Geometry: final body of the model. Coordinates: model frame, mm. Face numbers are marked on the shaded views. A direction names the side the tool comes from. Coordinates: 2 decimals unless noted, no trailing zeros. Loops run counter-clockwise (first coordinate to the right, second up) from the corner with the lowest first, then second, coordinate; pieces in that order, holes last. Notation, with made-up numbers: (-16.5, 26.25) - (3.5, 26.25) arc R22 cw to (3.5, 62.25) - close; hole circle Ø8 at (15, 46). An arc over 180 degrees is marked (long way). Put each result on its own line as item: value. Start each with the question number.
1) Section D-D on x = 33. Output: boundary loops of the cut face in (y, z).
2) Material intervals for line 1 along X through (y, z) = (-3, 0); line 2 along Y through (x, z) = (0, 420); line 3 along Z through (x, y) = (0, -7), sorted ascending. Write a range as from..to.
3) Section A-A on x = 0. Output: boundary loops of the cut face in (y, z).
4) Reachability of the marked faces 1, 2 and 3 from +Z, -Z, +X, -X, +Y, -Y: full face, straight path, thin tool, end or side. Return the list, or none.
5) Section C-C on y = 36. Output: boundary loops of the cut face in (x, z), and give its area (3 significant figures).
6) Section B-B on z = 0. Output: boundary loops of the cut face in (x, y), and give its area (3 significant figures).
7) Contact query for flat-ended pins moving along their axis: pin 1 Ø10 at (y, z) = (52.5, 105.5) entering from -X; pin 2 Ø12 at (y, z) = (-8.5, 409.5) entering from +X; pin 3 Ø2 at (x, z) = (9, 283) entering from -Y. Output: stop coordinate, or through.
```python
from build123d import *

# Parameters (mm, degrees)
SKETCH2_R               = 20
BOSS_EXTRUDE1_DEPTH     = 20
SKETCH3_R               = 63.245553203
SKETCH3_R_2             = 55
CUT_EXTRUDE1_DEPTH      = 101
CUT_EXTRUDE1_DEPTH_BACK = 10


with BuildPart() as part:
    # Sketch1 → Revolve1 (revolve)
    with BuildSketch(Plane(origin=(0, 0, 0), x_dir=(1, 0, 0), z_dir=(0, 1, 0))):
        Polygon((70, -600), (70, -550), (60, -550), (60, -40), (0, -40), (0, -60), (45, -60), (45, -520), (25, -520), (25, -600), align=None)
    revolve(axis=Axis((0, 0, 0), (0, 0, 1)))

    # Sketch2 → Boss-Extrude1 (add, symmetric)
    with BuildSketch(Plane(origin=(0, 0, 0), x_dir=(1, 0, 0), z_dir=(0, 1, 0))):
        with BuildLine():
            Line((60, -40), (60, 0))
            ThreePointArc((60, 0), (0, 60), (-60, 0))
            Line((-60, 0), (-60, -40))
            Line((-60, -40), (60, -40))
        make_face()
        Circle(SKETCH2_R, mode=Mode.SUBTRACT)
    extrude(amount=BOSS_EXTRUDE1_DEPTH, both=True)

    # Sketch3 → Cut-Extrude1 (cut, two sides)
    with BuildSketch(Plane(origin=(0, 0, 40), x_dir=(-1, 0, 0), z_dir=(0, 0, -1))) as cut_extrude1_sk:
        Circle(SKETCH3_R)
        Circle(SKETCH3_R_2, mode=Mode.SUBTRACT)
    extrude(amount=CUT_EXTRUDE1_DEPTH, mode=Mode.SUBTRACT)
    extrude(cut_extrude1_sk.sketch, amount=-CUT_EXTRUDE1_DEPTH_BACK, mode=Mode.SUBTRACT)


solid = part.part
```
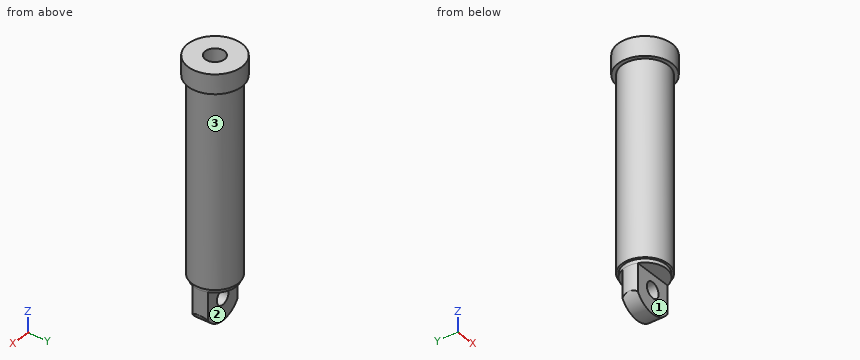
Answer block:
1. outline: (-61.73, 550) - (-50.11, 550) - (-50.11, 50) - (-44, 50) - (-44, 40) - (-20, 40) - (-20, -50.11) - (20, -50.11) - (20, 40) - (44, 40) - (44, 50) - (50.11, 50) - (50.11, 550) - (61.73, 550) - (61.73, 600) - (-61.73, 600) - close; hole (-30.59, 60) - (30.59, 60) - (30.59, 520) - (-30.59, 520) - close
2. line 1: x = -54.92..-20, 20..54.92
2. line 2: y = -60..-45, 45..60
2. line 3: z = -60..-20, 20..60
3. outline: (-70, 550) - (-60, 550) - (-60, 50) - (-55, 50) - (-55, 40) - (-20, 40) - (-20, 20) - (20, 20) - (20, 40) - (55, 40) - (55, 50) - (60, 50) - (60, 550) - (70, 550) - (70, 600) - (25, 600) - (25, 520) - (45, 520) - (45, 60) - (-45, 60) - (-45, 520) - (-25, 520) - (-25, 600) - (-70, 600) - close; (-20, -60) - (20, -60) - (20, -20) - (-20, -20) - close
4. face 1: -Z, +X, -X, -Y
4. face 2: -Z, +X, -X, +Y
4. face 3: -Z
5. outline: (-60.03, 550) - (-48, 550) - (-48, 50) - (-41.58, 50) - (-41.58, 40) - (41.58, 40) - (41.58, 50) - (48, 50) - (48, 550) - (60.03, 550) - (60.03, 600) - (-60.03, 600) - close; hole (-27, 60) - (27, 60) - (27, 520) - (-27, 520) - close
5. area: 30,000 mm²
6. outline: (-51.23, -20) - (-20, -20) - (-20, 20) - (-51.23, 20) arc R55 ccw to start; (20, -20) - (51.23, -20) arc R55 ccw to (51.23, 20) - (20, 20) - close
6. area: 2,700 mm²
7. pin 1: stops at x = -36.66
7. pin 2: stops at x = 59.95
7. pin 3: stops at y = -59.46
